For this review, take the finished solid that the model builds, in its own axes (mm). Round coordinates to 2 decimals unless told otherwise and drop trailing zeros. Loops run counter-clockwise (first coordinate to the right, second up) from the corner with the lowest first, then second, coordinate; pieces in that order, holes last.
1) Take a section at B-B (x = 18.25). State the section outline as (y, z) points, then the cut area to 3 significant figures.
2) Take a section at C-C (z = 16). State the section outline as (x, y) points, then the cut area to 3 significant figures.
3) Insertion check: pin 1 (4.5 mm diameter, centred on x = 0, z = 0, fed in from +Y); pin 2 (2 mm diameter, centred on y = 1.5, z = 13, fed in from +X); pin 3 (1.2 mm diameter, centred on x = 0, z = 13.25, fed in from -Y); pin 4 (2.5 mm diameter, centred on x = -13.25, z = 0, fed in from -Y). Each pin has a flat end and moves straight along its axis. Give the tip position at first contact, or say it passes through.
4) Wall thickness on L1, parallel to Y at x = 1.5, z = 16; L2, parallel to Z at x = -23.25, y = 3.8; L3, parallel to X at y = 2, z = 21.5: over which ranges is each line inside the solid? List them lowest first.
5) Mouldability with a two-part tool opening along X and no side actions: class faces 1 (the cylindrical face through (-0.04, 3.54, 19.25)), 2 (the cylindrical face through (-0.056, 3.535, -26.187)), 3 (the flat face through (3.725, 3.535, -15.972)), 4 (the flat face through (0, 3, -2)) as pulls with the +X half, pulls with the -X half, needs draft (parallel to the pull), parting line crosses it, or undercut.
6) Take a section at A-A (z = -13.25). State the section outline as (x, y) points.
7) Take a section at D-D (x = -15.5). State the section outline as (y, z) points, then the cut area to 3 significant figures.
```python
from build123d import *

# Parameters (mm, degrees)
ESQUISSE1_R                            = 9.25
ESQUISSE1_R_2                          = 1.65
BOSS_EXTRU_1_DEPTH                     = 8
BOSS_EXTRU_2_DEPTH                     = 8
R_P_TITION_CIRCULAIRE1_COUNT           = 4
ESQUISSE3_R                            = 1
ENL_V_MAT_EXTRU_1_DEPTH                = 8
R_P_TITION_LIN_AIRE1_COUNT             = 4
R_P_TITION_LIN_AIRE1_PITCH             = 5
R_P_TITION_CIRCULAIRE2_COUNT           = 4
R_P_TITION_CIRCULAIRE2_COPY_1_SKETCH_R = 1
R_P_TITION_CIRCULAIRE2_COPY_1_DEPTH    = 8
R_P_TITION_CIRCULAIRE2_COPY_2_SKETCH_R = 1
R_P_TITION_CIRCULAIRE2_COPY_2_DEPTH    = 8
R_P_TITION_CIRCULAIRE2_COPY_3_SKETCH_R = 1
R_P_TITION_CIRCULAIRE2_COPY_3_DEPTH    = 8
R_P_TITION_CIRCULAIRE2_COPY_4_SKETCH_R = 1
R_P_TITION_CIRCULAIRE2_COPY_4_DEPTH    = 8
R_P_TITION_CIRCULAIRE2_COPY_5_SKETCH_R = 1
R_P_TITION_CIRCULAIRE2_COPY_5_DEPTH    = 8
R_P_TITION_CIRCULAIRE2_COPY_6_SKETCH_R = 1
R_P_TITION_CIRCULAIRE2_COPY_6_DEPTH    = 8
R_P_TITION_CIRCULAIRE2_COPY_7_SKETCH_R = 1
R_P_TITION_CIRCULAIRE2_COPY_7_DEPTH    = 8
R_P_TITION_CIRCULAIRE2_COPY_8_SKETCH_R = 1
R_P_TITION_CIRCULAIRE2_COPY_8_DEPTH    = 8
R_P_TITION_CIRCULAIRE2_COPY_9_SKETCH_R = 1
R_P_TITION_CIRCULAIRE2_COPY_9_DEPTH    = 8
ESQUISSE4_W                            = 74.025208854
ESQUISSE4_H                            = 65.087506081
ESQUISSE4_R                            = 6
ENL_V_MAT_EXTRU_2_DEPTH                = 2
ESQUISSE5_R                            = 4
ENL_V_MAT_EXTRU_3_DEPTH                = 5
BOSS_EXTRU_3_DEPTH                     = 5
R_P_TITION_CIRCULAIRE3_COUNT           = 24
ESQUISSE7_R                            = 34.023023218
ESQUISSE7_R_2                          = 4.5
ENL_V_MAT_EXTRU_4_DEPTH                = 1
ESQUISSE8_R                            = 2.75
ENL_V_MAT_EXTRU_5_DEPTH                = 1
CHANFREIN1_SIZE                        = 1


with BuildPart() as part:
    # Esquisse1 → Boss.-Extru.1 (new body)
    with BuildSketch(Plane(origin=(0, 0, 0), x_dir=(1, 0, 0), z_dir=(0, 1, 0))):
        with Locations(Location((0, 0, 0), (0, 0, 270))):
            Circle(ESQUISSE1_R)
        with Locations(Location((0, 0, 0), (0, 0, 270))):
            Circle(ESQUISSE1_R_2, mode=Mode.SUBTRACT)
    extrude(amount=BOSS_EXTRU_1_DEPTH)

    # Esquisse2 → Boss.-Extru.2 (add)
    with BuildSketch(Plane(origin=(0, 8, 0), x_dir=(1, 0, 0), z_dir=(0, 1, 0))):
        with BuildLine():
            Line((-4.75, 7.937253933), (-2.7278844, 23.785315281))
            ThreePointArc((-2.7278844, 23.785315281), (0, 26.187253933), (2.7278844, 23.785315281))
            Line((2.7278844, 23.785315281), (4.75, 7.937253933))
            Line((4.75, 7.937253933), (-4.75, 7.937253933))
        make_face()
    boss_extru_2 = extrude(amount=-BOSS_EXTRU_2_DEPTH)

    # Répétition circulaire1: Boss.-Extru.2 ×4 about axis
    r_p_tition_circulaire1_axis = Axis((0, 0, 0), (0, 1, 0))
    for i in range(1, R_P_TITION_CIRCULAIRE1_COUNT):
        add(boss_extru_2.rotate(r_p_tition_circulaire1_axis, i * 360 / R_P_TITION_CIRCULAIRE1_COUNT))

    # Esquisse3 → Enlèv. mat.-Extru.1 (cut)
    with BuildSketch(Plane(origin=(0, 8, 0), x_dir=(1, 0, 0), z_dir=(0, 1, 0))):
        with Locations(Location((0, 8.25, 0), (0, 0, 270))):
            Circle(ESQUISSE3_R)
    enl_v_mat_extru_1 = extrude(amount=-ENL_V_MAT_EXTRU_1_DEPTH, mode=Mode.SUBTRACT)

    # Répétition linéaire1: Enlèv. mat.-Extru.1 ×4
    with Locations(*[(0, 0, -i * R_P_TITION_LIN_AIRE1_PITCH) for i in range(1, R_P_TITION_LIN_AIRE1_COUNT)]):
        add(enl_v_mat_extru_1, mode=Mode.SUBTRACT)

    # Répétition circulaire2: Enlèv. mat.-Extru.1 ×4 about axis
    r_p_tition_circulaire2_axis = Axis((0, 0, 0), (0, 1, 0))
    for i in range(1, R_P_TITION_CIRCULAIRE2_COUNT):
        add(enl_v_mat_extru_1.rotate(r_p_tition_circulaire2_axis, i * 360 / R_P_TITION_CIRCULAIRE2_COUNT), mode=Mode.SUBTRACT)

    # Répétition circulaire2 copy 1 sketch → Répétition circulaire2 copy 1 (cut)
    with BuildSketch(Plane(origin=(-5, 8, 0), x_dir=(0, 0, -1), z_dir=(0, 1, 0))):
        with Locations(Location((0, 8.25, 0), (0, 0, 270))):
            Circle(R_P_TITION_CIRCULAIRE2_COPY_1_SKETCH_R)
    extrude(amount=-R_P_TITION_CIRCULAIRE2_COPY_1_DEPTH, mode=Mode.SUBTRACT)

    # Répétition circulaire2 copy 2 sketch → Répétition circulaire2 copy 2 (cut)
    with BuildSketch(Plane(origin=(0, 8, 5), x_dir=(-1, 0, 0), z_dir=(0, 1, 0))):
        with Locations(Location((0, 8.25, 0), (0, 0, 270))):
            Circle(R_P_TITION_CIRCULAIRE2_COPY_2_SKETCH_R)
    extrude(amount=-R_P_TITION_CIRCULAIRE2_COPY_2_DEPTH, mode=Mode.SUBTRACT)

    # Répétition circulaire2 copy 3 sketch → Répétition circulaire2 copy 3 (cut)
    with BuildSketch(Plane(origin=(5, 8, 0), x_dir=(0, 0, 1), z_dir=(0, 1, 0))):
        with Locations(Location((0, 8.25, 0), (0, 0, 270))):
            Circle(R_P_TITION_CIRCULAIRE2_COPY_3_SKETCH_R)
    extrude(amount=-R_P_TITION_CIRCULAIRE2_COPY_3_DEPTH, mode=Mode.SUBTRACT)

    # Répétition circulaire2 copy 4 sketch → Répétition circulaire2 copy 4 (cut)
    with BuildSketch(Plane(origin=(-10, 8, 0), x_dir=(0, 0, -1), z_dir=(0, 1, 0))):
        with Locations(Location((0, 8.25, 0), (0, 0, 270))):
            Circle(R_P_TITION_CIRCULAIRE2_COPY_4_SKETCH_R)
    extrude(amount=-R_P_TITION_CIRCULAIRE2_COPY_4_DEPTH, mode=Mode.SUBTRACT)

    # Répétition circulaire2 copy 5 sketch → Répétition circulaire2 copy 5 (cut)
    with BuildSketch(Plane(origin=(0, 8, 10), x_dir=(-1, 0, 0), z_dir=(0, 1, 0))):
        with Locations(Location((0, 8.25, 0), (0, 0, 270))):
            Circle(R_P_TITION_CIRCULAIRE2_COPY_5_SKETCH_R)
    extrude(amount=-R_P_TITION_CIRCULAIRE2_COPY_5_DEPTH, mode=Mode.SUBTRACT)

    # Répétition circulaire2 copy 6 sketch → Répétition circulaire2 copy 6 (cut)
    with BuildSketch(Plane(origin=(10, 8, 0), x_dir=(0, 0, 1), z_dir=(0, 1, 0))):
        with Locations(Location((0, 8.25, 0), (0, 0, 270))):
            Circle(R_P_TITION_CIRCULAIRE2_COPY_6_SKETCH_R)
    extrude(amount=-R_P_TITION_CIRCULAIRE2_COPY_6_DEPTH, mode=Mode.SUBTRACT)

    # Répétition circulaire2 copy 7 sketch → Répétition circulaire2 copy 7 (cut)
    with BuildSketch(Plane(origin=(-15, 8, 0), x_dir=(0, 0, -1), z_dir=(0, 1, 0))):
        with Locations(Location((0, 8.25, 0), (0, 0, 270))):
            Circle(R_P_TITION_CIRCULAIRE2_COPY_7_SKETCH_R)
    extrude(amount=-R_P_TITION_CIRCULAIRE2_COPY_7_DEPTH, mode=Mode.SUBTRACT)

    # Répétition circulaire2 copy 8 sketch → Répétition circulaire2 copy 8 (cut)
    with BuildSketch(Plane(origin=(0, 8, 15), x_dir=(-1, 0, 0), z_dir=(0, 1, 0))):
        with Locations(Location((0, 8.25, 0), (0, 0, 270))):
            Circle(R_P_TITION_CIRCULAIRE2_COPY_8_SKETCH_R)
    extrude(amount=-R_P_TITION_CIRCULAIRE2_COPY_8_DEPTH, mode=Mode.SUBTRACT)

    # Répétition circulaire2 copy 9 sketch → Répétition circulaire2 copy 9 (cut)
    with BuildSketch(Plane(origin=(15, 8, 0), x_dir=(0, 0, 1), z_dir=(0, 1, 0))):
        with Locations(Location((0, 8.25, 0), (0, 0, 270))):
            Circle(R_P_TITION_CIRCULAIRE2_COPY_9_SKETCH_R)
    extrude(amount=-R_P_TITION_CIRCULAIRE2_COPY_9_DEPTH, mode=Mode.SUBTRACT)

    # Esquisse4 → Enlèv. mat.-Extru.2 (cut)
    with BuildSketch(Plane(origin=(0, 8, 0), x_dir=(1, 0, 0), z_dir=(0, 1, 0))):
        with Locations((-0.052574722, -0.420597777)):
            Rectangle(ESQUISSE4_W, ESQUISSE4_H)
        with Locations(Location((0, 0, 0), (0, 0, 270))):
            Circle(ESQUISSE4_R, mode=Mode.SUBTRACT)
    extrude(amount=-ENL_V_MAT_EXTRU_2_DEPTH, mode=Mode.SUBTRACT)

    # Esquisse5 → Enlèv. mat.-Extru.3 (cut)
    with BuildSketch(Plane(origin=(0, 8, 0), x_dir=(1, 0, 0), z_dir=(0, 1, 0))):
        with Locations(Location((0, 0, 0), (0, 0, 270))):
            Circle(ESQUISSE5_R)
    extrude(amount=-ENL_V_MAT_EXTRU_3_DEPTH, mode=Mode.SUBTRACT)

    # Esquisse6 → Boss.-Extru.3 (add)
    with BuildSketch(Plane(origin=(0, 8, 0), x_dir=(1, 0, 0), z_dir=(0, 1, 0))):
        Polygon((-0.3, 4), (-0.139230485, 3.4), (0.139230485, 3.4), (0.3, 4), align=None)
    boss_extru_3 = extrude(amount=-BOSS_EXTRU_3_DEPTH)

    # Répétition circulaire3: Boss.-Extru.3 ×24 about axis
    r_p_tition_circulaire3_axis = Axis((0, 0, 0), (0, 1, 0))
    for i in range(1, R_P_TITION_CIRCULAIRE3_COUNT):
        add(boss_extru_3.rotate(r_p_tition_circulaire3_axis, i * 360 / R_P_TITION_CIRCULAIRE3_COUNT))

    # Esquisse7 → Enlèv. mat.-Extru.4 (cut)
    with BuildSketch(Plane.XZ):
        Circle(ESQUISSE7_R)
        with Locations(Location((0, 0, 0), (0, 0, 270))):
            Circle(ESQUISSE7_R_2, mode=Mode.SUBTRACT)
    extrude(amount=-ENL_V_MAT_EXTRU_4_DEPTH, mode=Mode.SUBTRACT)

    # Esquisse8 → Enlèv. mat.-Extru.5 (cut)
    with BuildSketch(Plane.XZ):
        with Locations(Location((0, 0, 0), (0, 0, 270))):
            Circle(ESQUISSE8_R)
    extrude(amount=-ENL_V_MAT_EXTRU_5_DEPTH, mode=Mode.SUBTRACT)

    # Chanfrein1
    chanfrein1_edges = [part.edges().sort_by_distance(p)[0] for p in [
        (0, 1, 4.5),
    ]]
    chamfer(chanfrein1_edges, length=CHANFREIN1_SIZE - 0.0001)  # a hair under: the kernel refuses the full size


solid = part.part
```
Response:
1. outline: (1, -3.43) - (6, -3.43) - (6, -1) - (1, -1) - close; (1, 1) - (6, 1) - (6, 3.43) - (1, 3.43) - close
1. area: 24.3 mm2
2. outline: (-3.72, 1) - (3.72, 1) - (3.72, 6) - (-3.72, 6) - close
2. area: 37.2 mm2
3. pin 1: stops at y = 3
3. pin 2: stops at x = 4.23
3. pin 3: passes through
3. pin 4: stops at y = 1
4. L1: y = 1 to 6
4. L2: z = -2.8 to -1, 1 to 2.8
4. L3: x = -3.02 to 3.02
5. face 1: undercut
5. face 2: parting line crosses it
5. face 3: pulls with the +X half
5. face 4: undercut
6. outline: (-4.07, 1) - (-1, 1) - (-1, 6) - (-4.07, 6) - close; (1, 1) - (4.07, 1) - (4.07, 6) - (1, 6) - close
7. outline: (1, -3.79) - (6, -3.79) - (6, 3.79) - (1, 3.79) - close
7. area: 37.9 mm2
